The drawing under review shows one solid part. Ordinate dimensions are in mm from its lowest x, y, z. A direction names the side the tool comes from. Round coordinates to 2 decimals unless told otherwise and drop trailing zeros. Order: outer loops, then holes, each group sorted by start corner. A loop starts at its lowest first (then second) coordinate and runs counter-clockwise, first axis right, second up.
1) Machinability: for the marked faces 1 and 2, which of the approach directions +Z, -Z, +X, -X, +Y, -Y give a long, thin tool a straight path to every point of the face, cutting with its end or side? Answer none if there is none.
2) Consider section D-D (y = 9.5). Give the boundary of the cut face in (x, z), then the cut area to 3 significant figures.
3) Clearance check with flat-ended pins moving along their axes: P1, Ø3, axis at x = 4, z = 6.5, coming from the -Y side; P2, Ø1, axis at x = 52.5, y = 3.5, coming from the -Z side; P3, Ø2.5, axis at x = 54.5, z = 5, coming from the -Y side (3 decimals); P4, Ø0.8, axis at x = 31.5, z = 20.5, coming from the +Y side. State where each tip first meets the part, or that it passes through.
4) Consider section A-A (x = 5). Give the boundary of the cut face in (y, z), then the cut area to 3 significant figures.
5) To check wall thickness, follow L1, parallel to X at y = 23.4, z = 15; L2, parallel to Y at x = 5, z = 20.65; L3, parallel to Z at x = 5, y = 23.3. State the ranges of each line that lie inside material, in increasing order.
6) Consider section C-C (z = 15). Give the boundary of the cut face in (x, y), then the cut area to 3 significant figures.
7) Consider section B-B (y = 5). Give the boundary of the cut face in (x, z).
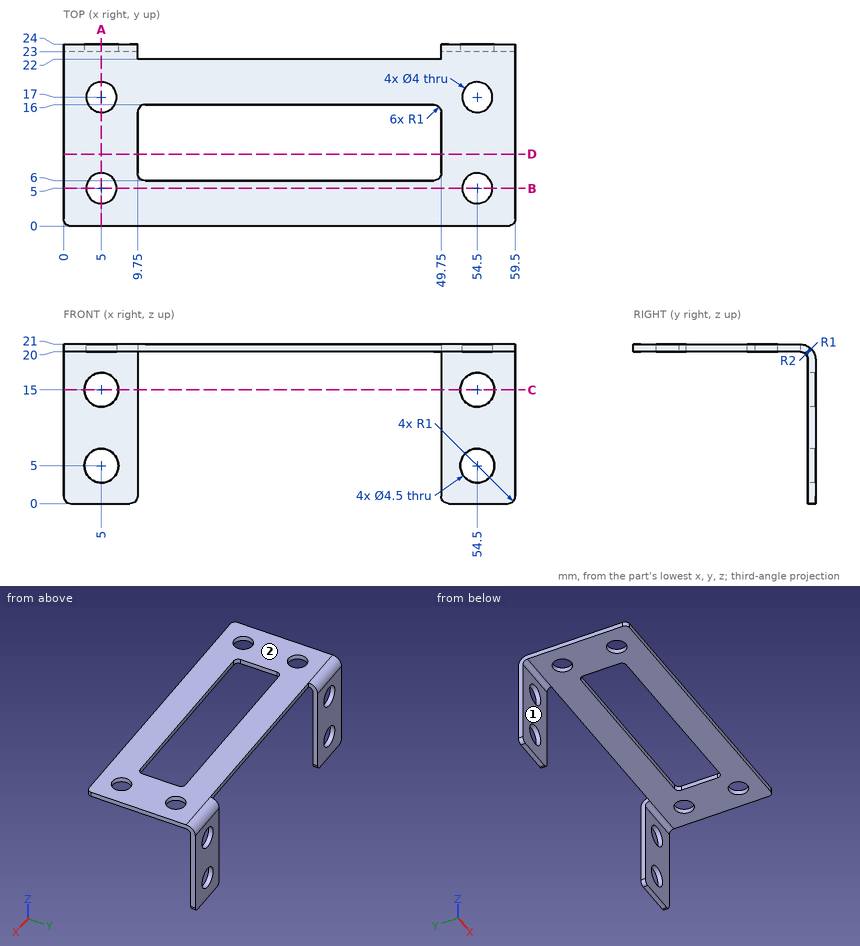
Answer below:
1. face 1: -Z, +X, -X, -Y
1. face 2: +Z, +X, -X, +Y, -Y
2. outline: (0, 20) - (9.75, 20) - (9.75, 21) - (0, 21) - close; (49.75, 20) - (59.5, 20) - (59.5, 21) - (49.75, 21) - close
2. area: 19.5 mm2
3. P1: stops at y = 23
3. P2: stops at z = 20
3. P3: passes through
3. P4: stops at y = 22
4. outline: (0, 20) - (3, 20) - (3, 21) - (0, 21) - close; (7, 20) - (15, 20) - (15, 21) - (7, 21) - close; (19, 20) - (22, 20) arc R1 cw to (23, 19) - (23, 17.25) - (24, 17.25) - (24, 19) arc R2 ccw to (22, 21) - (19, 21) - close; (23, 0) - (24, 0) - (24, 2.75) - (23, 2.75) - close; (23, 7.25) - (24, 7.25) - (24, 12.75) - (23, 12.75) - close
4. area: 26.4 mm2
5. L1: x = 0 to 2.75, 7.25 to 9.75, 49.75 to 52.25, 56.75 to 59.5
5. L2: y = 0 to 3, 7 to 15, 19 to 23.13
5. L3: z = 0 to 2.75, 7.25 to 12.75, 17.25 to 20.52
6. outline: (0, 23) - (2.75, 23) - (2.75, 24) - (0, 24) - close; (7.25, 23) - (9.75, 23) - (9.75, 24) - (7.25, 24) - close; (49.75, 23) - (52.25, 23) - (52.25, 24) - (49.75, 24) - close; (56.75, 23) - (59.5, 23) - (59.5, 24) - (56.75, 24) - close
6. area: 10.5 mm2
7. outline: (0, 20) - (3, 20) - (3, 21) - (0, 21) - close; (7, 20) - (52.5, 20) - (52.5, 21) - (7, 21) - close; (56.5, 20) - (59.5, 20) - (59.5, 21) - (56.5, 21) - close
